Could you check a few things on this drawing? It's one solid part, dimensions in mm from its lowest x, y, z. Round coordinates to 2 decimals unless told otherwise and drop trailing zeros. Write each loop counter-clockwise with the first axis right and the second up, starting at its lowest first coordinate (ties: lowest second). Pieces come first, ordered by that corner, then holes. Notation, with made-up numbers: (-13, 83) -> (11, 83) arc R19 ccw to (11, 106) -> close; hole circle Ø4 at (40.25, 22.5). An arc over 180 degrees is marked (long way). Answer in a Markdown table with one row per item. Add a question column.
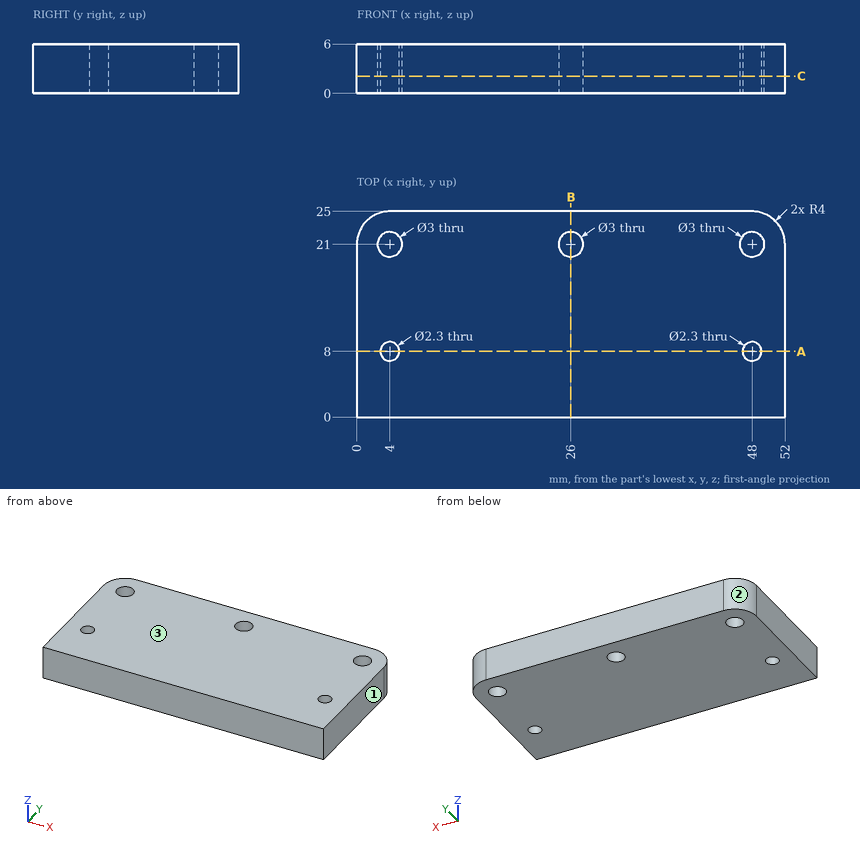
(1) If we mould it in two halves opening along X, with no side actions, what happens to the marked faces 1, 2 and 3? For each: pulls with the +X half, pulls with the -X half, needs draft (parallel to the pull), parting line crosses it, or undercut.
(2) Suppose I cut it at A-A, the plane y = 8. Please give me the cut outline in (x, z), then the cut area to 3 significant figures.
(3) I need wall thicknesses on L1, parallel to Y at x = 4, z = 4.65; L2, parallel to X at y = 20.5, z = 3.6; L3, parallel to X at y = 9, z = 5.65. Which ranges of each line are inside material? Lowest first, please.
(4) Suppose I cut it at C-C, the plane z = 2.1. Please give me the cut outline in (x, y).
(5) Suppose I cut it at B-B, the plane x = 26. Please give me the cut outline in (y, z).
(6) For P1, Ø1.8, axis at x = 48, y = 21, coming from the +Z side; P2, Ø4, axis at x = 26, y = 21, coming from the +Z side, each with a flat end and sliding along its axis, tell me the tip position at first contact or that it passes through.
Response:
| question | item | result |
|---|---|---|
| 1 | face 1 | pulls with the +X half |
| 1 | face 2 | pulls with the -X half |
| 1 | face 3 | needs draft |
| 2 | outline | (0, 0) -> (2.85, 0) -> (2.85, 6) -> (0, 6) -> close; (5.15, 0) -> (46.85, 0) -> (46.85, 6) -> (5.15, 6) -> close; (49.15, 0) -> (52, 0) -> (52, 6) -> (49.15, 6) -> close |
| 2 | area | 284 mm² |
| 3 | L1 | 0 to 6.85, 9.15 to 19.5, 22.5 to 25 |
| 3 | L2 | 0 to 2.59, 5.41 to 24.59, 27.41 to 46.59, 49.41 to 52 |
| 3 | L3 | 0 to 3.43, 4.57 to 47.43, 48.57 to 52 |
| 4 | outline | (0, 0) -> (52, 0) -> (52, 21) arc R4 ccw to (48, 25) -> (4, 25) arc R4 ccw to (0, 21) -> close; hole circle Ø3 at (4, 21); hole circle Ø2.3 at (4, 8); hole circle Ø3 at (26, 21); hole circle Ø3 at (48, 21); hole circle Ø2.3 at (48, 8) |
| 5 | outline | (0, 0) -> (19.5, 0) -> (19.5, 6) -> (0, 6) -> close; (22.5, 0) -> (25, 0) -> (25, 6) -> (22.5, 6) -> close |
| 6 | P1 | through |
| 6 | P2 | z = 6 |
